Could you check a few things on this model? Use its own coordinates, in mm. Face numbers are marked on the shaded views. A direction names the side the tool comes from. Round coordinates to 2 decimals unless told otherwise and drop trailing zeros. Loops run counter-clockwise (first coordinate to the right, second up) from the corner with the lowest first, then second, coordinate; pieces in that order, holes last. Notation, with made-up numbers: (-35, 47.25) - (-2, 47.25) arc R35 cw to (-2, 82.25) - close; hole circle Ø6 at (74, -17). An arc over 180 degrees is marked (long way). Use one line per item in the form item = value.
```python
from build123d import *

# Parameters (mm, degrees)
SKETCH1_W           = 11.5
SKETCH1_H           = 11.5
BOSS_EXTRUDE1_DEPTH = 69
BOSS_EXTRUDE2_START = -5.75
SKETCH3_W           = 11.5
SKETCH3_H           = 11.5
BOSS_EXTRUDE2_DEPTH = 100


with BuildPart() as part:
    # Sketch1 → Boss-Extrude1 (new body)
    with BuildSketch(Plane.XY):
        Rectangle(SKETCH1_W, SKETCH1_H)
    extrude(amount=BOSS_EXTRUDE1_DEPTH)

    # Sketch3 → Boss-Extrude2 (add)
    with BuildSketch(Plane(origin=(0, 0, 0), x_dir=(1, 0, 0), z_dir=(0, 1, 0)).offset(BOSS_EXTRUDE2_START)):
        with Locations((0, 5.75)):
            Rectangle(SKETCH3_W, SKETCH3_H)
    extrude(amount=BOSS_EXTRUDE2_DEPTH)


solid = part.part
```
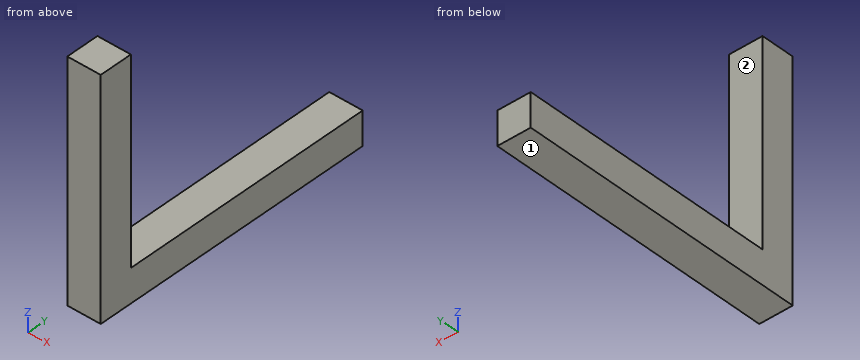
1. If we section it at A-A, the plane x = 3.25: Write out the boundary of the cut face in (y, z), plus the area to 3 significant figures.
Solution:
outline = (-5.75, -11.5) - (94.25, -11.5) - (94.25, 0) - (5.75, 0) - (5.75, 69) - (-5.75, 69) - close
area = 1,940 mm^2
2. Please list where these lines run through material, in increasing order: line 1 along Y through (x, z) = (2.75, 18.5); line 2 along Z through (x, y) = (-4.5, 50).
Solution:
line_1 = -5.75 to 5.75
line_2 = -11.5 to 0
3. For P1, Ø3.5, axis at x = -1, y = 45.5, coming from the +Z side; P2, Ø4, axis at x = -4, z = 40, coming from the +Y side, each with a flat end and sliding along its axis, tell me the tip position at first contact or that it passes through.
Solution:
P1 = 0
P2 = 5.75
4. If we section it at B-B, the plane z = 37: Write out the boundary of the cut face in (x, y).
Solution:
outline = (-5.75, -5.75) - (5.75, -5.75) - (5.75, 5.75) - (-5.75, 5.75) - close
5. If we section it at C-C, the plane y = 69: Write out the boundary of the cut face in (x, z), plus the area to 3 significant figures.
Solution:
outline = (-5.75, -11.5) - (5.75, -11.5) - (5.75, 0) - (-5.75, 0) - close
area = 132 mm^2
6. On a 3-axis mill with a long thin cutter (end or side, diameter ignored), from which of +Z, -Z, +X, -X, +Y, -Y can I reach the whole of each face in a straight line? I mean the marked faces 1 and 2. Say none if no direction works.
Solution:
face_1 = -Z, +X, -X, +Y, -Y
face_2 = +Z, +X, -X, +Y
